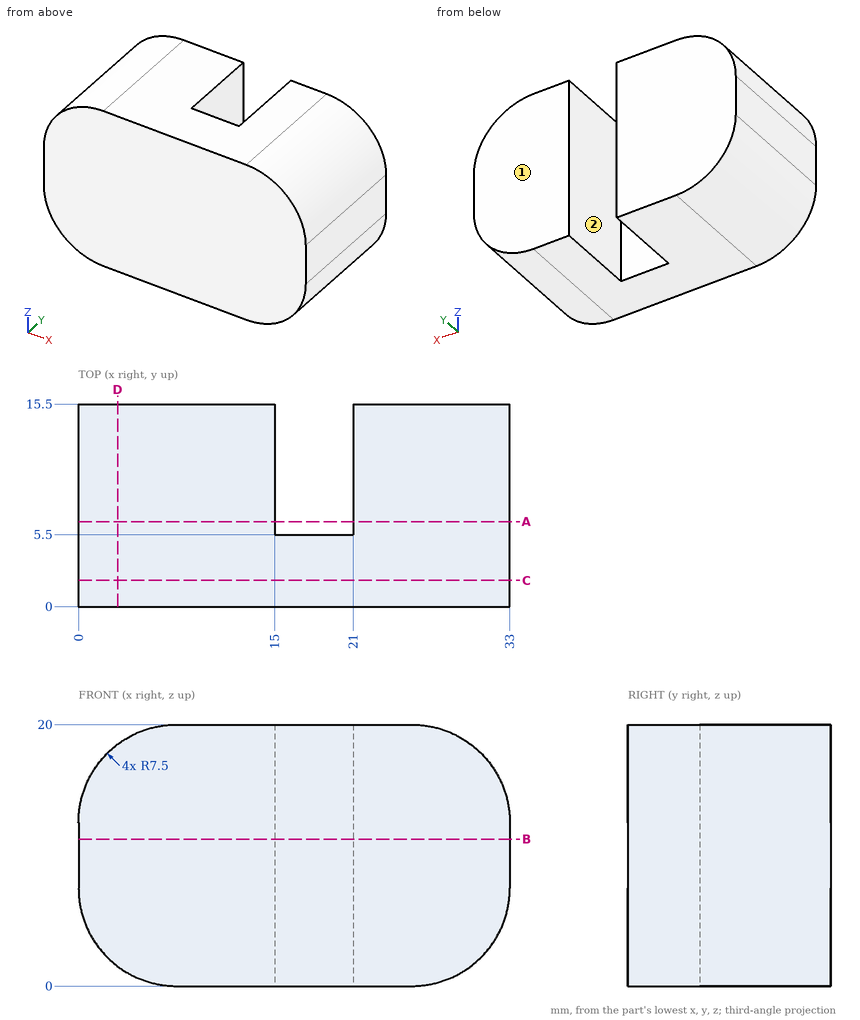
Geometry: see drawing. Coordinates: mm, zero at the bounding-box minimum. A direction names the side the tool comes from. Give positions to 0.01 mm unless a question says otherwise; leave off trailing zeros. Order: outer loops, then holes, each group sorted by start corner. A loop starts at its lowest first (then second) coordinate and runs counter-clockwise, first axis right, second up.
1. Cut plane D-D (x = 3). Return loops of the section in (y, z), and give its area (4 significant figures).
Computed:
outline: (0, 1.5) - (15.5, 1.5) - (15.5, 18.5) - (0, 18.5) - close
area: 263.5 mm2
2. Cut plane B-B (z = 11.25). Return loops of the section in (x, y).
Computed:
outline: (0, 0) - (33, 0) - (33, 15.5) - (21, 15.5) - (21, 5.5) - (15, 5.5) - (15, 15.5) - (0, 15.5) - close
3. Set-up query: the marked faces 1 and 2. Return all of +Z, -Z, +X, -X, +Y, -Y with unobstructed straight access to the full face (end or side cutting, diameter ignored); none if empty.
Computed:
face 1: +Z, -Z, +X, -X, +Y
face 2: +Z, -Z, +Y
4. Pin query (flat end, axial travel): pin 1 Ø5 at (x, y) = (29.5, 6.5) entering from +Z. Return the tip coordinate at first contact, or that it passes through.
Computed:
pin 1: stops at z = 19.85
5. Cut plane A-A (y = 6.5). Return loops of the section in (x, z), and give its area (3 significant figures).
Computed:
outline: (0, 7.5) arc R7.5 ccw to (7.5, 0) - (15, 0) - (15, 20) - (7.5, 20) arc R7.5 ccw to (0, 12.5) - close; (21, 0) - (25.5, 0) arc R7.5 ccw to (33, 7.5) - (33, 12.5) arc R7.5 ccw to (25.5, 20) - (21, 20) - close
area: 492 mm2
6. Cut plane C-C (y = 2). Return loops of the section in (x, z), and give its area (3 significant figures).
Computed:
outline: (0, 7.5) arc R7.5 ccw to (7.5, 0) - (25.5, 0) arc R7.5 ccw to (33, 7.5) - (33, 12.5) arc R7.5 ccw to (25.5, 20) - (7.5, 20) arc R7.5 ccw to (0, 12.5) - close
area: 612 mm2
7. Line query: probe 1 along X at (y, z) = (8, 8.5); probe 2 along X at (y, z) = (6, 4.75); probe 3 along Z at (x, y) = (6, 8). Output: solid intervals per line, ascending.
Computed:
probe 1: x = 0 to 15, 21 to 33
probe 2: x = 0.52 to 15, 21 to 32.48
probe 3: z = 0.15 to 19.85
